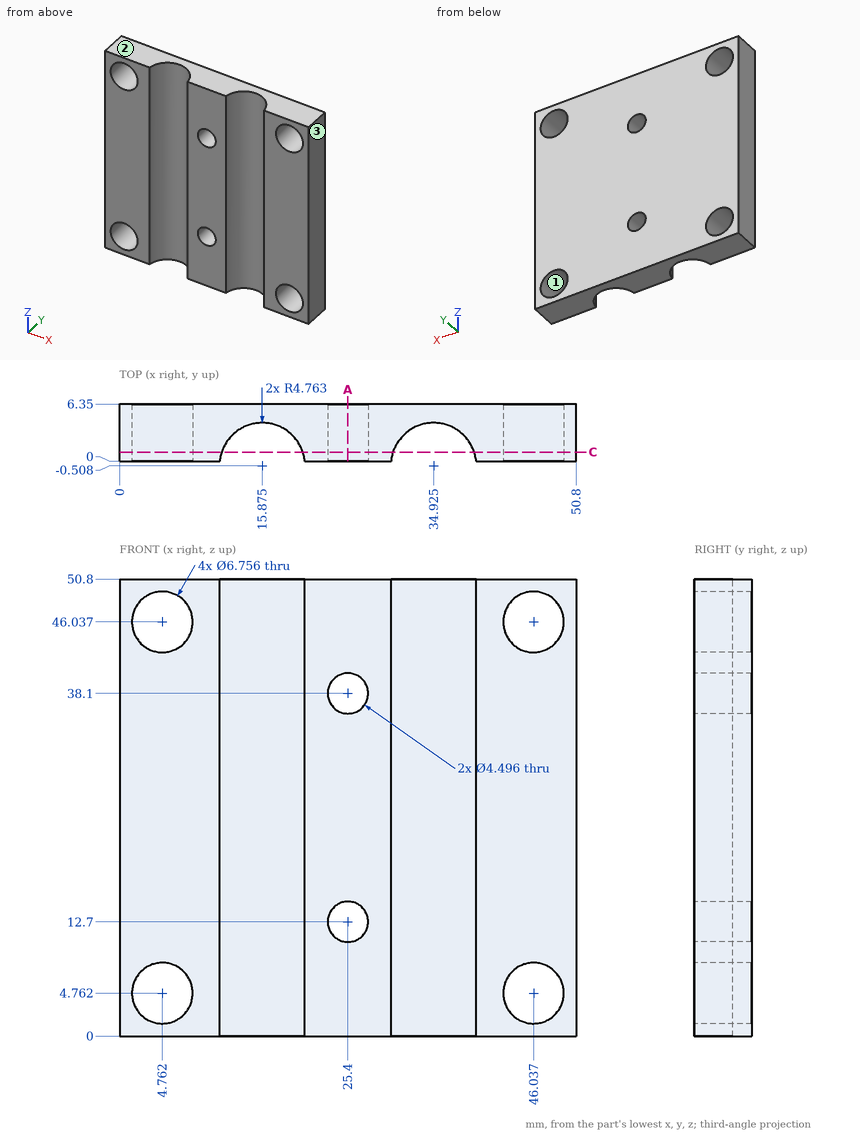
Design review of the part shown in the three views and the two pictorial views. Dimensions are in mm from the part's minimum x, y and z. Give positions to 0.01 mm unless a question says otherwise; leave off trailing zeros. Write each loop counter-clockwise with the first axis right and the second up, starting at its lowest first coordinate (ties: lowest second). Pieces come first, ordered by that corner, then holes.
Item 1: Take a section at C-C (y = 1). Give the number of separate pieces and of enclosed holes in the cut face, and give its area (3 significant figures).
Item 2: Take a section at A-A (x = 25.4). Give the boundary of the cut face in (y, z).
Item 3: Insertion check: P1, Ø8, axis at x = 4.76, z = 46.04, coming from the +Y side. The pin has a flat end and moves straight along its axis. Give the tip position at first contact, or say it passes through.
Item 4: Wall thickness on probe 1 along Z at (x, y) = (25.4, 5.25); probe 2 along Z at (x, y) = (46, 5.25) (1 decimal): over which ranges is each line inside the solid? List them lowest first.
Item 5: The part is to be moulded in two halves that separate along Z. For the marked faces 1, 2 and 3, say which applies: +Z half, -Z half, draft (parallel to the pull), parting line (faces both ways), or undercut.
Established:
1. separate pieces: 3
1. enclosed holes: 6
1. area: 1,490 mm2
2. outline: (0, 0) - (6.35, 0) - (6.35, 10.45) - (0, 10.45) - close; (0, 14.95) - (6.35, 14.95) - (6.35, 35.85) - (0, 35.85) - close; (0, 40.35) - (6.35, 40.35) - (6.35, 50.8) - (0, 50.8) - close
3. P1: stops at y = 6.35
4. probe 1: z = 0 to 10.45, 14.95 to 35.85, 40.35 to 50.8
4. probe 2: z = 0 to 1.4, 8.1 to 42.7, 49.4 to 50.8
5. face 1: undercut
5. face 2: +Z half
5. face 3: draft
